Work out the finished part from the listing and answer in its coordinate system (mm). Face numbers are marked on the shaded views. A direction names the side the tool comes from. Round coordinates to 2 decimals unless told otherwise and drop trailing zeros. Write each loop counter-clockwise with the first axis right and the second up, starting at its lowest first coordinate (ties: lowest second). Pieces come first, ordered by that corner, then holes. Notation, with made-up numbers: (-6, 13) - (46, 13) arc R23 cw to (46, 32) - close; hole circle Ø3 at (-8, -30.5). An arc over 180 degrees is marked (long way). Write item = value, one per line. Start each with the question number.
from build123d import *

# Parameters (mm, degrees)
SKETCH_R      = 2.5
PAD_DEPTH     = 2
SKETCH001_R   = 19
PAD001_DEPTH  = 2
SKETCH002_R   = 6.5
SKETCH002_R_2 = 4.5
PAD002_DEPTH  = 26
SKETCH003_R   = 28
PAD003_DEPTH  = 33


with BuildPart() as part:
    # Sketch → Pad (new body, symmetric)
    with BuildSketch(Plane.XY):
        with BuildLine():
            ThreePointArc((19.641791, 19.95495), (0, 28), (-19.641791, 19.95495))
            Line((-36.656716, 3.207046), (-19.641791, 19.95495))
            ThreePointArc((-36.656716, 3.207046), (-38, 0), (-36.656716, -3.207046))
            Line((-36.656716, -3.207046), (-19.641791, -19.95495))
            ThreePointArc((-19.641791, -19.95495), (0, -28), (19.641791, -19.95495))
            Line((36.656716, -3.207046), (19.641791, -19.95495))
            ThreePointArc((36.656716, -3.207046), (38, 0), (36.656716, 3.207046))
            Line((19.641791, 19.95495), (36.656716, 3.207046))
        make_face()
        with Locations((-33.5, 0)):
            Circle(SKETCH_R, mode=Mode.SUBTRACT)
        with Locations((33.5, 0)):
            Circle(SKETCH_R, mode=Mode.SUBTRACT)
        with Locations((24.5, 0)):
            Circle(SKETCH_R, mode=Mode.SUBTRACT)
        with Locations((-24.5, 0)):
            Circle(SKETCH_R, mode=Mode.SUBTRACT)
        with Locations((0, 25)):
            Circle(SKETCH_R, mode=Mode.SUBTRACT)
        with Locations((0, -25)):
            Circle(SKETCH_R, mode=Mode.SUBTRACT)
    extrude(amount=PAD_DEPTH, both=True)

    # Sketch001 → Pad001 (new body)
    with BuildSketch(Plane.XY.offset(2)):
        with Locations((-0.290907, -0.018148)):
            Circle(SKETCH001_R)
    extrude(amount=PAD001_DEPTH)

    # Sketch002 → Pad002 (new body)
    with BuildSketch(Plane.XY.offset(4)):
        Circle(SKETCH002_R)
        Circle(SKETCH002_R_2, mode=Mode.SUBTRACT)
    extrude(amount=PAD002_DEPTH)

    # Sketch003 → Pad003 (new body)
    with BuildSketch(Plane(origin=(0, 0, -2), x_dir=(1, 0, 0), z_dir=(0, 0, -1))):
        with Locations((-0.396294, -0.105837)):
            Circle(SKETCH003_R)
    extrude(amount=PAD003_DEPTH)


solid = part.part
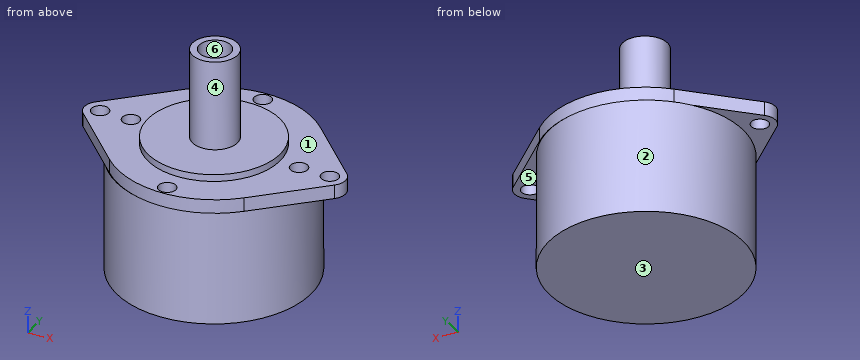
1. Find section B-B on y = 9. Give the vertices of the cut face in (x, z), plus the area to 3 significant figures.
2. Each of these flat-tipped pins is pushed along its axis until it touches: pin 1 (10 mm diameter, centred on x = 3.5, y = -11.5, fed in from +Z); pin 2 (3 mm diameter, centred on x = -13.5, y = -24.5, fed in from +Z); pin 3 (10 mm diameter, centred on x = -13.5, z = -16, fed in from +Y). Where does it stop, or does it pass through?
3. Find section C-C on x = 1. Give the vertices of the cut face in (y, z).
4. Find section A-A on x = -33.5. Give the vertices of the cut face in (y, z), plus the area to 3 significant figures.
5. For a pull along X with two mould halves and no side action, classify the marked faces 4, 5 and 6 as released by +X, released by -X, zero draft, split by the parting line, or undercut.
6. Which of the six approach directions +Z, -Z, +X, -X, +Y, -Y give full straight-line access (tool end or side, diameter ignored) to the marked faces 1, 2 and 3?
7. Find section D-D on z = 25.5. Give the vertices of the cut face in (x, y).
8. Consider line 1 (Y direction, x = 0, z = -1.1); line 2 (X direction, y = 0.5, z = -15.5); line 3 (Z direction, x = 14.5, y = -4). Determine where each line is inside the solid, lowest interval first.
Answer key:
q1.outline = (-30.77, -2) - (-26.95, -2) - (-26.95, -35) - (26.15, -35) - (26.15, -2) - (30.77, -2) - (30.77, 2) - (16.43, 2) - (16.43, 4) - (-17.01, 4) - (-17.01, 2) - (-30.77, 2) - close
q1.area = 2,070 mm²
q2.pin_1 = 4
q2.pin_2 = 2
q2.pin_3 = 26.91
q3.outline = (-27.98, -2) - (-27.86, -2) - (-27.86, -35) - (28.07, -35) - (28.07, -2) - (27.98, -2) - (27.98, 2) - (27.29, 2) - (27.29, -2) - (22.71, -2) - (22.71, 2) - (18.94, 2) - (18.94, 4) - (6.42, 4) - (6.42, 30) - (4.39, 30) - (4.39, 4) - (-4.39, 4) - (-4.39, 30) - (-6.42, 30) - (-6.42, 4) - (-18.97, 4) - (-18.97, 2) - (-22.71, 2) - (-22.71, -2) - (-27.29, -2) - (-27.29, 2) - (-27.98, 2) - close
q4.outline = (-6.31, -2) - (-2.5, -2) - (-2.5, 2) - (-6.31, 2) - close; (2.5, -2) - (6.31, -2) - (6.31, 2) - (2.5, 2) - close
q4.area = 30.5 mm²
q5.face_4 = split by the parting line
q5.face_5 = zero draft
q5.face_6 = undercut
q6.face_1 = +Z
q6.face_2 = -Z
q6.face_3 = -Z, +X, -X, +Y, -Y
q7.outline = circle Ø13 at (0, 0); hole circle Ø9 at (0, 0)
q8.line_1 = -28 to -27.5, -22.5 to 22.5, 27.5 to 28
q8.line_2 = -28.39 to 27.6
q8.line_3 = -35 to 4
